Model file for the job. Use its own axes, mm. Round coordinates to 2 decimals unless told otherwise and drop trailing zeros. Loops run counter-clockwise (first coordinate to the right, second up) from the corner with the lowest first, then second, coordinate; pieces in that order, holes last. Notation, with made-up numbers: M 67.25,-34.5 L 87.25,-34.5 A28 cw 87.25,2.5 Z; hole C 27.25,48.5 d3. An arc over 180 degrees is marked long. Answer in a Markdown table with one row per item.
from build123d import *

# Parameters (mm, degrees)
SKETCH_1_W      = 100.2
SKETCH_1_H      = 100
SKETCH_1_R      = 3.14
SKETCH_1_R_2    = 2
EXTRUDE_1_DEPTH = 5
FILLET_1_R      = 10


with BuildPart() as part:
    # 草图1 → 凸台-拉伸1 (new body)
    with BuildSketch(Plane(origin=(0, 0, 0), x_dir=(1, 0, 0), z_dir=(0, 1, 0))):
        with Locations((4.40209205, 20.757531381)):
            Rectangle(SKETCH_1_W, SKETCH_1_H)
        with Locations(Location((-19.64790795, 55.307531381, 0), (0, 0, 270))):
            Circle(SKETCH_1_R, mode=Mode.SUBTRACT)
        with Locations(Location((28.45209205, 55.307531381, 0), (0, 0, 270))):
            Circle(SKETCH_1_R, mode=Mode.SUBTRACT)
        with Locations(Location((28.45209205, -13.792468619, 0), (0, 0, 270))):
            Circle(SKETCH_1_R, mode=Mode.SUBTRACT)
        with Locations(Location((-19.64790795, -13.792468619, 0), (0, 0, 270))):
            Circle(SKETCH_1_R, mode=Mode.SUBTRACT)
        with Locations(Location((-19.64790795, 65.110023284, 0), (0, 0, 270))):
            Circle(SKETCH_1_R_2, mode=Mode.SUBTRACT)
        with Locations(Location((4.40209205, 65.110023284, 0), (0, 0, 270))):
            Circle(SKETCH_1_R_2, mode=Mode.SUBTRACT)
        with Locations(Location((28.45209205, 65.110023284, 0), (0, 0, 270))):
            Circle(SKETCH_1_R_2, mode=Mode.SUBTRACT)
        with Locations(Location((28.45209205, -23.594960523, 0), (0, 0, 90))):
            Circle(SKETCH_1_R_2, mode=Mode.SUBTRACT)
        with Locations(Location((4.40209205, -23.594960523, 0), (0, 0, 90))):
            Circle(SKETCH_1_R_2, mode=Mode.SUBTRACT)
        with Locations(Location((-19.64790795, -23.594960523, 0), (0, 0, 90))):
            Circle(SKETCH_1_R_2, mode=Mode.SUBTRACT)
    extrude(amount=EXTRUDE_1_DEPTH)

    # 圆角1
    fillet_1_edges = [part.edges().sort_by_distance(p)[0] for p in [
        (-45.69790795, 2.5, -70.757531381),
        (54.50209205, 2.5, -70.757531381),
        (54.50209205, 2.5, 29.242468619),
        (-45.69790795, 2.5, 29.242468619),
    ]]
    fillet(fillet_1_edges, radius=FILLET_1_R)


solid = part.part
1. Pin check, flat tip, straight feed: pin 1 (5.5 mm diameter, centred on x = -19.65, z = -55.31, fed in from +Y). Stop position of the tip, or through.
Verdict:
| item | result |
|---|---|
| pin 1 | passes through |
2. Wall check: probe 1 along X at (y, z) = (4.7, 16.5); probe 2 along X at (y, z) = (0.5, -65); probe 3 along Z at (x, y) = (6, 4.7). Give the ranges that are in metal, low to high.
Verdict:
| item | result |
|---|---|
| probe 1 | x = -45.7 to -21.24, -18.06 to 26.86, 30.04 to 54.5 |
| probe 2 | x = -44.75 to -21.64, -17.65 to 2.41, 6.4 to 26.46, 30.45 to 53.56 |
| probe 3 | z = -70.76 to -66.31, -63.91 to 22.39, 24.8 to 29.24 |
3. Saw through at A-A (z = 12). Write the cut outline in (x, y).
Verdict:
| item | result |
|---|---|
| outline | M -45.7,0 L -22.23,0 L -22.23,5 L -45.7,5 Z; M -17.07,0 L 25.87,0 L 25.87,5 L -17.07,5 Z; M 31.03,0 L 54.5,0 L 54.5,5 L 31.03,5 Z |
4. Mould opens along X. For faces 1 (the cylindrical face through (-42.846, 2.535, 26.235)), 2 (the cylindrical face through (-17, 2.46, 15.48)), 3 (the flat face through (4, 2, 29.242)) say: +X half, -X half, draft (parallel to the pull), parting line (faces both ways), or undercut.
Verdict:
| item | result |
|---|---|
| face 1 | -X half |
| face 2 | undercut |
| face 3 | draft |
5. Saw through at B-B (y = 3.25). State how many separate pieces and enclosed holes the cut face has, and give its area (3 significant figures).
Verdict:
| item | result |
|---|---|
| separate pieces | 1 |
| enclosed holes | 10 |
| area | 9,730 mm² |
